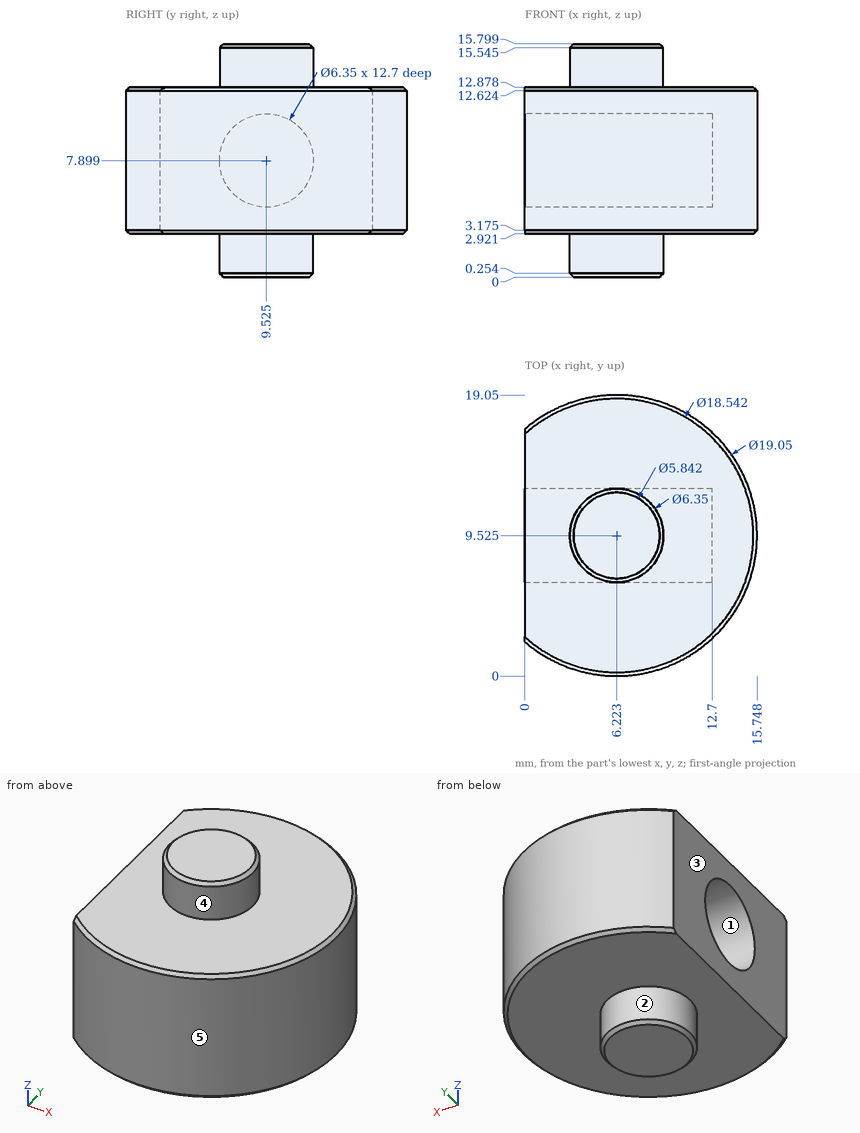
Geometry: see drawing. Coordinates: mm, zero at the bounding-box minimum. A direction names the side the tool comes from. Round coordinates to 2 decimals unless told otherwise and drop trailing zeros. Use CSV: the item, a comma, the result in double quotes.
(1) Ray query, L1, parallel to Z at x = 2.5, y = 14; L2, parallel to Y at x = 8.25, z = 10.25; L3, parallel to Y at x = 8.5, z = 5.25 (1 decimal). Return the intervals inside material, ascending.
Report:
L1,"2.92 to 12.88"
L2,"0.22 to 7.39, 11.66 to 18.83"
L3,"0.3 to 7.8, 11.3 to 18.8"
(2) Access query for the marked faces 4 and 5. Directions: +Z, -Z, +X, -X, +Y, -Y. A direction counts if a zero-diameter tool reaches every point of the face in a straight line with its end or side. Return the directions, or none.
Report:
face 4,"+Z"
face 5,"+Z, -Z"
(3) First-contact query: pin 1 Ø6 at (x, z) = (8.5, 8.5) entering from -Y; pin 2 Ø6 at (x, y) = (4, 2.5) entering from -Z; pin 3 Ø3 at (y, z) = (9, 8.5) entering from -X; pin 4 Ø1.5 at (x, y) = (2, 6) entering from +Z. Flat tips, straight axial feed; report the tip coordinate or a pass-through.
Report:
pin 1,"y = 0"
pin 2,"z = 2.92"
pin 3,"x = 12.7"
pin 4,"z = 12.88"
(4) Pull-direction query (Y, two-part tool) for the marked faces 1, 2 and 3; classes: +Y half, -Y half, draft (parallel to the pull), parting line (faces both ways), or undercut.
Report:
face 1,"undercut"
face 2,"parting line"
face 3,"draft"
